```python
from build123d import *

# Parameters (mm, degrees)
SKIZZE1_W                        = 35
SKIZZE1_H                        = 75
AUFSATZ_LINEAR_AUSTRAGEN1_DEPTH  = 1.5
SKIZZE3_W                        = 15.25
SKIZZE3_H                        = 5
SKIZZE3_W_2                      = 4.875
SCHNITT_LINEAR_AUSTRAGEN12_DEPTH = 20
SCHNITT_LINEAR_AUSTRAGEN18_DEPTH = 1.5
SKIZZE14_W                       = 1
SKIZZE14_H                       = 57.312152727
AUFSATZ_LINEAR_AUSTRAGEN2_DEPTH  = 1.5


with BuildPart() as part:
    # Skizze1 → Aufsatz-Linear austragen1 (new body)
    with BuildSketch(Plane.XY):
        with Locations((17.5, 37.5)):
            Rectangle(SKIZZE1_W, SKIZZE1_H)
    extrude(amount=AUFSATZ_LINEAR_AUSTRAGEN1_DEPTH)

    # Skizze3 → Schnitt-Linear austragen12 (cut)
    with BuildSketch(Plane.XY.offset(1.5)):
        with Locations((17.5, 2.5)):
            Rectangle(SKIZZE3_W, SKIZZE3_H)
        with Locations((32.5625, 2.5)):
            Rectangle(SKIZZE3_W_2, SKIZZE3_H)
        with Locations((2.4375, 2.5)):
            Rectangle(SKIZZE3_W_2, SKIZZE3_H)
    extrude(amount=-SCHNITT_LINEAR_AUSTRAGEN12_DEPTH, mode=Mode.SUBTRACT)

    # Skizze13 → Schnitt-Linear austragen18 (cut)
    with BuildSketch(Plane.XY.offset(1.5)):
        with BuildLine():
            ThreePointArc((21.674459995, 40.249493876), (17.5, 63.500000179), (13.325540005, 40.249493876))
            ThreePointArc((13.325540005, 40.249493876), (17.5, 17.000948841), (21.674459995, 40.249493876))
        make_face()
        with BuildLine():
            Line((15.117508566, 40.761111111), (15.117508566, 39.738888889))
            ThreePointArc((15.117508566, 39.738888889), (17.5, 18), (19.882491434, 39.738888889))
            Line((19.882491434, 39.738888889), (19.882491434, 40.761111111))
            ThreePointArc((19.882491434, 40.761111111), (17.5, 62.5), (15.117508566, 40.761111111))
        make_face(mode=Mode.SUBTRACT)
    extrude(amount=-SCHNITT_LINEAR_AUSTRAGEN18_DEPTH, mode=Mode.SUBTRACT)


with BuildPart() as schnitt_linear_austragen18_piece_1:
    # of the separate pieces the step leaves, piece 1, a body of its own (schnitt_linear_austragen18_pieces)
    add(part.part.solids().sort_by_distance((4.875, 0, 0))[0])



with BuildPart() as schnitt_linear_austragen18_piece_2:
    # of the separate pieces the step leaves, piece 2, a body of its own (schnitt_linear_austragen18_pieces)
    add(part.part.solids().sort_by_distance((19.882491434, 39.738888889, 0))[0])


with BuildPart() as schnitt_linear_austragen18_piece_1_1:
    add(schnitt_linear_austragen18_piece_1.part)

    add(schnitt_linear_austragen18_piece_2.part)  # Aufsatz-Linear austragen2 merges Schnitt-Linear austragen18 piece 2
    # Skizze14 → Aufsatz-Linear austragen2 (add)
    with BuildSketch(Plane.XY.offset(1.5)):
        with Locations((17.5, 39.529651928)):
            Rectangle(SKIZZE14_W, SKIZZE14_H)
    extrude(amount=-AUFSATZ_LINEAR_AUSTRAGEN2_DEPTH)


solid = schnitt_linear_austragen18_piece_1_1.part
```
Geometry: final body of the model. Coordinates: model frame, mm. A direction names the side the tool comes from. Give positions to 0.01 mm unless a question says otherwise; leave off trailing zeros. Write each loop counter-clockwise with the first axis right and the second up, starting at its lowest first coordinate (ties: lowest second). Pieces come first, ordered by that corner, then holes.
1. Line query: probe 1 along X at (y, z) = (51, 0.75); probe 2 along X at (y, z) = (38, 0.8); probe 3 along Y at (x, z) = (15, 1.45). Output: solid intervals per line, ascending.
2. Section query B-B, the plane z = 0.65. Return loops of the section in (x, y) (1 decimal).
3. Reachability of faces 4 (the flat face through (2, 5, 1)), 5 (the flat face through (17, 5, 1)), 6 (the flat face through (30.125, 2, 1)), 7 (the cylindrical face through (29.314, 26.899, 0.76)) from +Z, -Z, +X, -X, +Y, -Y: full face, straight path, thin tool, end or side. Return the list, or none.
4. Section query A-A, the plane y = 35. Return loops of the section in (x, z), then the cut area to 3 significant figures.
5. Section query C-C, the plane x = 3. Return loops of the section in (y, z).
6. Section query D-D, the plane y = 59. Return loops of the section in (x, z), then the cut area to 3 significant figures.
7. Pin query (flat end, axial travel): P1, Ø1, axis at x = 13.5, y = 19, coming from the -Z side; P2, Ø0.8, axis at x = 16.5, z = 1, coming from the -Y side. Return the tip coordinate at first contact, or that it passes through.
8. Draft query along Y for faces 1 (the flat face through (33, 5, 1)), 2 (the cylindrical face through (28.438, 27.83, 0.76)), 3 (the flat face through (9.875, 2, 1)). Return one class per face: released by +Y, released by -Y, zero draft, split by the parting line, or undercut.
Computed:
1. probe 1: x = 0 to 5.51, 6.51 to 28.49, 29.49 to 35
1. probe 2: x = 0 to 9.56, 11.18 to 23.82, 25.44 to 35
1. probe 3: y = 5 to 17.26, 18.29 to 39.71, 40.79 to 62.21, 63.24 to 75
2. outline: (0, 5) - (4.9, 5) - (4.9, 0) - (9.9, 0) - (9.9, 5) - (25.1, 5) - (25.1, 0) - (30.1, 0) - (30.1, 5) - (35, 5) - (35, 75) - (0, 75) - close; hole (13.3, 40.2) arc R12 ccw to (17, 17) - (17, 18) arc R11 cw to (15.1, 39.7) - (15.1, 40.8) arc R11 cw to (17, 62.5) - (17, 63.5) arc R12 ccw to start; hole (18, 17) arc R12 ccw to (21.7, 40.2) arc R12 ccw to (18, 63.5) - (18, 62.5) arc R11 cw to (19.9, 40.8) - (19.9, 39.7) arc R11 cw to (18, 18) - close
3. face 4: +Z, -Z, -X, -Y
3. face 5: +Z, -Z, -Y
3. face 6: +Z, -Z, +X, -Y
3. face 7: +Z, -Z
4. outline: (0, 0) - (7.11, 0) - (7.11, 1.5) - (0, 1.5) - close; (8.28, 0) - (26.72, 0) - (26.72, 1.5) - (8.28, 1.5) - close; (27.89, 0) - (35, 0) - (35, 1.5) - (27.89, 1.5) - close
4. area: 49.0 mm2
5. outline: (5, 0) - (75, 0) - (75, 1.5) - (5, 1.5) - close
6. outline: (0, 0) - (8.13, 0) - (8.13, 1.5) - (0, 1.5) - close; (9.45, 0) - (25.55, 0) - (25.55, 1.5) - (9.45, 1.5) - close; (26.87, 0) - (35, 0) - (35, 1.5) - (26.87, 1.5) - close
6. area: 48.5 mm2
7. P1: stops at z = 0
7. P2: stops at y = 5
8. face 1: released by -Y
8. face 2: undercut
8. face 3: zero draft
